Input: part model. Units: mm. Frame: model coordinates. Coordinates: 2 decimals unless noted, no trailing zeros. Write each loop counter-clockwise with the first axis right and the second up, starting at its lowest first coordinate (ties: lowest second). Pieces come first, ordered by that corner, then holes. Notation, with made-up numbers: (4, 75) - (16, 75) arc R14 ccw to (16, 81) - close; hole circle Ø8 at (48, 14). An arc over 180 degrees is marked (long way). Use a Markdown table: item, result. Add a question column.
Q1. Mould query, pull axis Z, two halves, no side actions, for faces 1 (the face through (1.972, 6.572, 5.938)), 2 (the face through (1.972, -5.878, 5.938)), 3 (the face through (3, 0, 15)), 4 (the face through (3, 0, 0)). Classes: released by +Z, released by -Z, zero draft, split by the parting line, or undercut.
Q2. Section query A-A (z = 7.5). Return the cut outline in (x, y) (3 decimals), then the cut area to 3 significant figures.
Q3. Section query B-B (x = 0.6). Return the cut outline in (y, z) (3 decimals).
Q4. Material intervals for probe 1 along Y at (x, z) = (0.9, 5.5); probe 2 along Y at (x, z) = (2.2, 13.25); probe 3 along Z at (x, y) = (3.55, 6), sorted ascending. Write a range as from..to.
Q5. Section query C-C (z = 1.5). Return the cut outline in (x, y), then the cut area to 3 significant figures.
Q6. Section query D-D (x = 3.1). Return the cut outline in (y, z) (3 decimals).
from build123d import *

# Parameters (mm, degrees)
F1_DEPTH = 15
F3_DEPTH = 25
F4_R     = 1.6
F5_DEPTH = 25


with BuildPart() as f1:
    # F0 (on Top) → F1 (new body)
    with BuildSketch(Plane.XY):
        with BuildLine():
            ThreePointArc((0, 4), (2.8284271247, 2.8284271247), (4, 0))
            Line((4, 0), (4, 10))
            Line((4, 10), (0, 10))
            Line((0, 10), (0, 4))
        make_face()
        with BuildLine():
            Line((4, -10), (4, 0))
            ThreePointArc((4, 0), (2.8284271247, -2.8284271247), (0, -4))
            Line((0, -4), (0, -10))
            Line((0, -10), (4, -10))
        make_face()
        with BuildLine():
            ThreePointArc((0, 2.45), (1.7324116139, 1.7324116139), (2.45, 0))
            Line((2.45, 0), (4, 0))
            ThreePointArc((4, 0), (2.8284271247, 2.8284271247), (0, 4))
            Line((0, 4), (0, 2.45))
        make_face()
        with BuildLine():
            Line((4, 0), (2.45, 0))
            ThreePointArc((2.45, 0), (1.7324116139, -1.7324116139), (0, -2.45))
            Line((0, -2.45), (0, -4))
            ThreePointArc((0, -4), (2.8284271247, -2.8284271247), (4, 0))
        make_face()
    extrude(amount=F1_DEPTH)

    # F2 (on face) → F3 (cut)
    with BuildSketch(Plane(origin=(0, 0, 0), x_dir=(0, -1, 0), z_dir=(-1, 0, 0))):
        with BuildLine():
            ThreePointArc((4.625, 7.5), (6.225, 5.9), (7.825, 7.5))
            Line((7.825, 7.5), (4.625, 7.5))
        make_face()
        with BuildLine():
            Line((4.625, 7.5), (7.825, 7.5))
            ThreePointArc((7.825, 7.5), (6.225, 9.1), (4.625, 7.5))
        make_face()
    extrude(amount=-F3_DEPTH, mode=Mode.SUBTRACT)

    # F4 (on face) → F5 (cut)
    with BuildSketch(Plane(origin=(0, 0, 0), x_dir=(0, -1, 0), z_dir=(-1, 0, 0))):
        with Locations((-6.225, 7.5)):
            Circle(F4_R)
    extrude(amount=-F5_DEPTH, mode=Mode.SUBTRACT)


solid = f1.part
Values follow:
| question | item | result |
|---|---|---|
| 1 | face 1 | undercut |
| 1 | face 2 | undercut |
| 1 | face 3 | released by +Z |
| 1 | face 4 | released by -Z |
| 2 | outline | (0, -10) - (4, -10) - (4, -7.825) - (0, -7.825) - close; (0, -4.625) - (4, -4.625) - (4, 4.625) - (0, 4.625) - (0, 2.45) arc R2.45 cw to (0, -2.45) - close; (0, 7.825) - (4, 7.825) - (4, 10) - (0, 10) - close |
| 2 | area | 45.0 mm2 |
| 3 | outline | (-10, 0) - (-2.375, 0) - (-2.375, 15) - (-10, 15) - close; (2.375, 0) - (10, 0) - (10, 15) - (2.375, 15) - close; hole circle Ø3.2 at (-6.225, 7.5); hole circle Ø3.2 at (6.225, 7.5) |
| 4 | probe 1 | -10..-2.28, 2.28..10 |
| 4 | probe 2 | -10..-1.08, 1.08..10 |
| 4 | probe 3 | 0..5.92, 9.08..15 |
| 5 | outline | (0, -10) - (4, -10) - (4, 10) - (0, 10) - (0, 2.45) arc R2.45 cw to (0, -2.45) - close |
| 5 | area | 70.6 mm2 |
| 6 | outline | (-10, 0) - (10, 0) - (10, 15) - (-10, 15) - close; hole circle Ø3.2 at (-6.225, 7.5); hole circle Ø3.2 at (6.225, 7.5) |
